Source: three-view drawing plus pictorial views. Frame: mm from the lowest corner of the part. A direction names the side the tool comes from. Coordinates: 2 decimals unless noted, no trailing zeros. Write each loop counter-clockwise with the first axis right and the second up, starting at its lowest first coordinate (ties: lowest second). Pieces come first, ordered by that corner, then holes. Notation, with made-up numbers: (71, 43) - (118, 43) arc R27 ccw to (118, 75) - close; hole circle Ø2 at (-30, 48). An arc over 180 degrees is marked (long way). One line per item, written item: value.
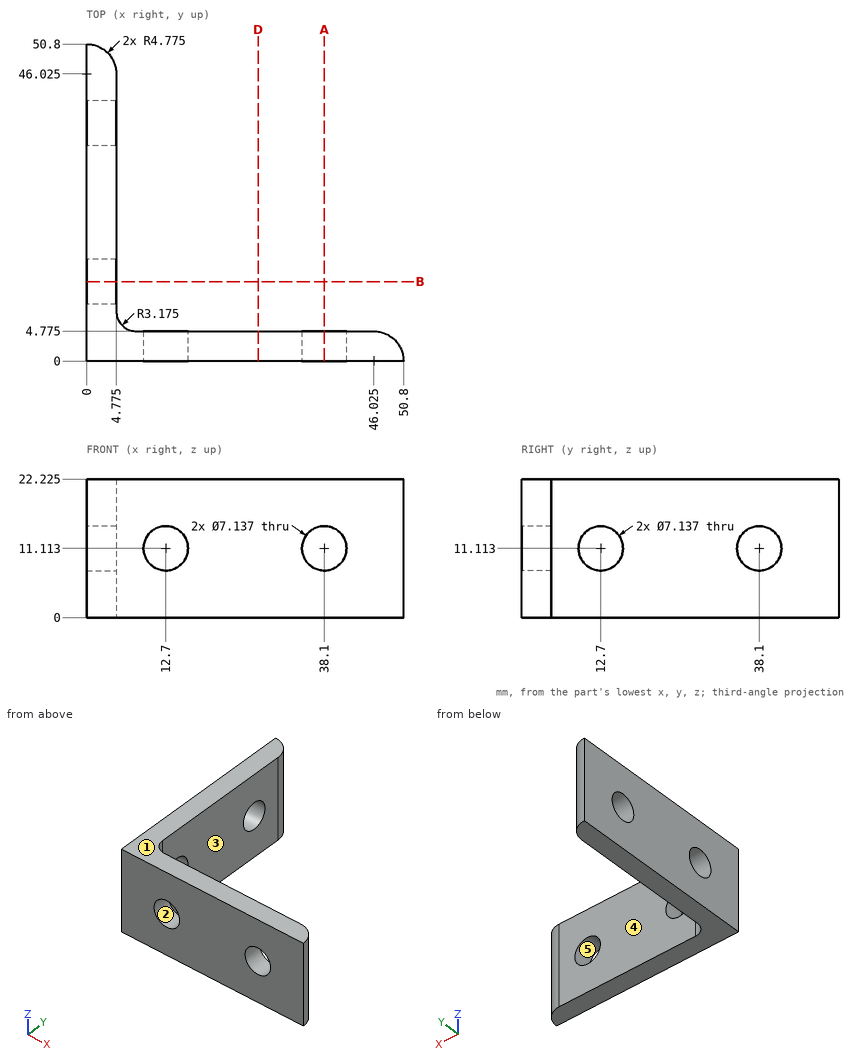
1) Reachability of the marked faces 4 and 5 from +Z, -Z, +X, -X, +Y, -Y: full face, straight path, thin tool, end or side. Return the list, or none.
Values found:
face 4: +Z, -Z, +X, +Y
face 5: +Y, -Y
2) Section query A-A on x = 38.1. Output: boundary loops of the cut face in (y, z) (1 decimal).
Values found:
outline: (0, 0) - (4.8, 0) - (4.8, 7.5) - (0, 7.5) - close; (0, 14.7) - (4.8, 14.7) - (4.8, 22.2) - (0, 22.2) - close
3) Material intervals for line 1 (Z direction, x = 2, y = 38) (1 decimal); line 2 (Y direction, x = 4, z = 12.5) (1 decimal); line 3 (Y direction, x = 17, z = 3.75) (1 decimal), sorted ascending.
Values found:
line 1: 0 to 7.5, 14.7 to 22.2
line 2: 0 to 9.4, 16 to 34.8, 41.4 to 48.6
line 3: 0 to 4.8
4) Section query D-D on x = 27.5. Output: boundary loops of the cut face in (y, z) (1 decimal), then the cut area to 3 significant figures.
Values found:
outline: (0, 0) - (4.8, 0) - (4.8, 22.2) - (0, 22.2) - close
area: 106 mm2
5) Contact query for flat-ended pins moving along their axis: P1, Ø12, axis at y = 38, z = 16, coming from the +X side (1 decimal); P2, Ø6.5, axis at x = 34, z = 15, coming from the +Y side (1 decimal). Output: stop coordinate, or through.
Values found:
P1: x = 4.8
P2: y = 4.8
6) Draft query along Z for the marked faces 1, 2 and 3. Return one class per face: released by +Z, released by -Z, zero draft, split by the parting line, or undercut.
Values found:
face 1: released by +Z
face 2: undercut
face 3: zero draft
